Could you check a few things on this drawing? It's one solid part, dimensions in mm from its lowest x, y, z. A direction names the side the tool comes from. Coordinates: 2 decimals unless noted, no trailing zeros. Loops run counter-clockwise (first coordinate to the right, second up) from the corner with the lowest first, then second, coordinate; pieces in that order, holes last. Notation, with made-up numbers: M -36,-30.5 L 14,-30.5 A20 ccw 14,-14.5 Z; hole C 39,17.25 d8. An arc over 180 degrees is marked long. Answer as a JSON object with one key per item and string values. Group by question number.
Item 1: Suppose I cut it at D-D (z = 1.5). Write out the boundary of the cut face in (x, y) (1 decimal).
Item 2: Suppose I cut it at A-A (z = 8). Write out the boundary of the cut face in (x, y) (1 decimal).
Item 3: If I drill on line 1 (Z direction, x = 5, y = 20.9); line 2 (X direction, y = 10, z = 11.5); line 3 (X direction, y = 12, z = 8.5), over which ranges is the centre line in solid material (lowest first)?
Item 4: I'm going to push flat-ended pins straight in: pin 1 Ø1.5 at (y, z) = (14.5, 12) entering from -X; pin 2 Ø2.5 at (y, z) = (1, 9) entering from +X; pin 3 Ø11 at (x, y) = (20, 10) entering from -Z; pin 4 Ø3.5 at (x, z) = (4.5, 8.5) entering from -Y. Where does each tip first touch, or does it pass through?
Item 5: Suppose I cut it at C-C (y = 5). Write out the boundary of the cut face in (x, z), then the cut area to 3 significant figures.
Item 6: Which directions (+Z, -Z, +X, -X, +Y, -Y) give clear straight access to the entire face, cutting with the end or side of a thin tool? Please do the marked faces 1, 2 and 3.
Item 7: Suppose I cut it at B-B (x = 5). Write out the boundary of the cut face in (y, z), then the cut area to 3 significant figures.
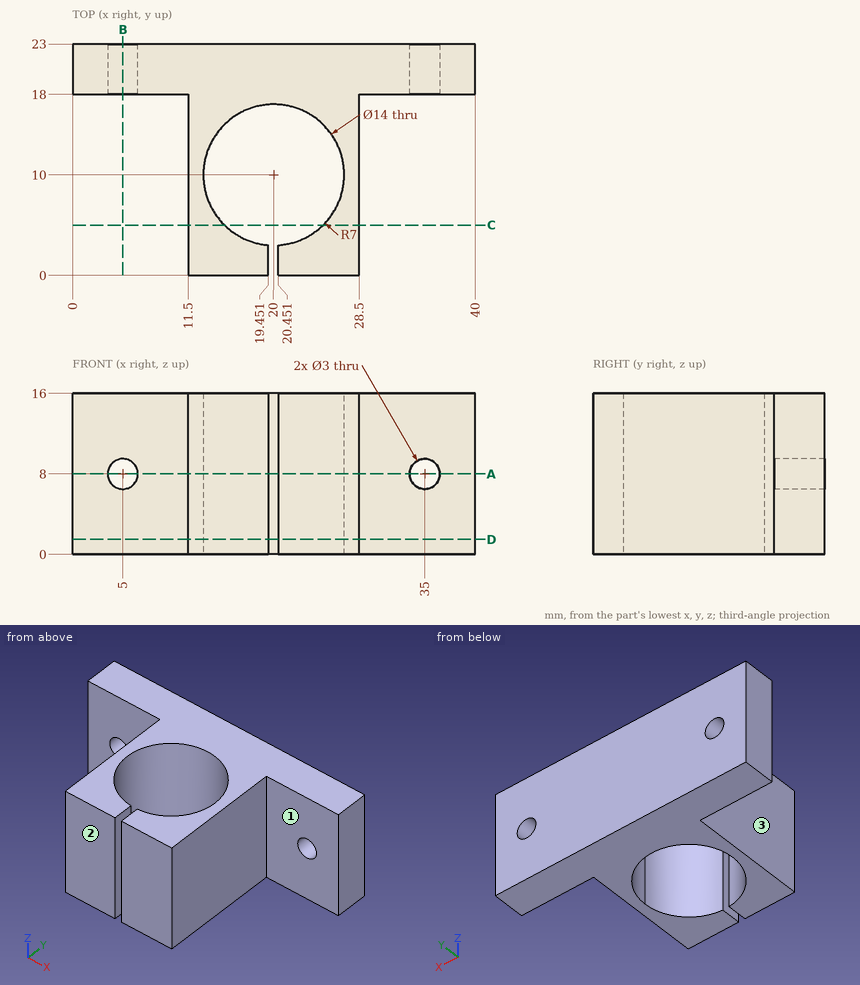
From the geometry:
{
 "1": {"outline": "M 0,18 L 11.5,18 L 11.5,0 L 19.5,0 L 19.5,3 A7 cw long 20.5,3 L 20.5,0 L 28.5,0 L 28.5,18 L 40,18 L 40,23 L 0,23 Z"},
 "2": {"outline": "M 0,18 L 3.5,18 L 3.5,23 L 0,23 Z; M 6.5,18 L 11.5,18 L 11.5,0 L 19.5,0 L 19.5,3 A7 cw long 20.5,3 L 20.5,0 L 28.5,0 L 28.5,18 L 33.5,18 L 33.5,23 L 6.5,23 Z; M 36.5,18 L 40,18 L 40,23 L 36.5,23 Z"},
 "3": {"line 1": "0 to 6.5, 9.5 to 16", "line 2": "11.5 to 13, 27 to 28.5", "line 3": "11.5 to 13.29, 26.71 to 28.5"},
 "4": {"pin 1": "x = 11.5", "pin 2": "x = 28.5", "pin 3": "through", "pin 4": "y = 18"},
 "5": {"outline": "M 11.5,0 L 15.1,0 L 15.1,16 L 11.5,16 Z; M 24.9,0 L 28.5,0 L 28.5,16 L 24.9,16 Z", "area": "115 mm2"},
 "6": {"face 1": "+Z, -Z, +X, -Y", "face 2": "+Z, -Z, +X, -X, -Y", "face 3": "+Z, -Z, -X, -Y"},
 "7": {"outline": "M 18,0 L 23,0 L 23,6.5 L 18,6.5 Z; M 18,9.5 L 23,9.5 L 23,16 L 18,16 Z", "area": "65.0 mm2"}
}
